The figure shows three views and two pictorial views of one solid part (mm, origin at its lowest corner). Answer the questions. A direction names the side the tool comes from. Coordinates: 2 decimals unless noted, no trailing zeros. Loops run counter-clockwise (first coordinate to the right, second up) from the corner with the lowest first, then second, coordinate; pieces in that order, holes last. Notation, with made-up numbers: M 60,9 L 108,9 A11 cw 108,30 Z; hole C 88,14.25 d4. An arc over 180 degrees is marked long. Answer as a JSON object with one key per item and string values. Group by question number.
1. Given pin 1 (5 mm diameter, centred on y = 39.05, z = 13.5, fed in from -X); pin 2 (1.8 mm diameter, centred on y = 43.05, z = 13.5, fed in from +X); pin 3 (3 mm diameter, centred on x = 5, z = 5.5, fed in from -Y), each flat-ended and moving along its own axis, determine where each tip first touches the part or whether it passes through.
2. A cutting plane is placed at D-D on x = 0.65. State how many separate pieces and enclosed holes the cut face has.
3. Determine the mould class of the marked faces 4, 5 and 6 for opening direction Y: released by +Y, released by -Y, zero draft, split by the parting line, or undercut.
4. A cutting plane is placed at B-B on y = 9.5. Give the vertices of the cut face in (x, z).
5. Straight lines are drawn through the part: L1, parallel to Z at x = 3.55, y = 14; L2, parallel to Y at x = 1.25, z = 6.25; L3, parallel to Z at x = 2.3, y = 20.5 (1 decimal). For each, find the intervals that lie inside material, in ascending order.
6. For the marked faces 1, 2 and 3, determine the directions among +Z, -Z, +X, -X, +Y, -Y from which every point of the face is accessible in a straight line to the end or side of a thin tool.
7. A cutting plane is placed at C-C on z = 13.5. Give the vertices of the cut face in (x, y).
8. A cutting plane is placed at A-A on z = 17.5. Give the vertices of the cut face in (x, y), and give its area (3 significant figures).
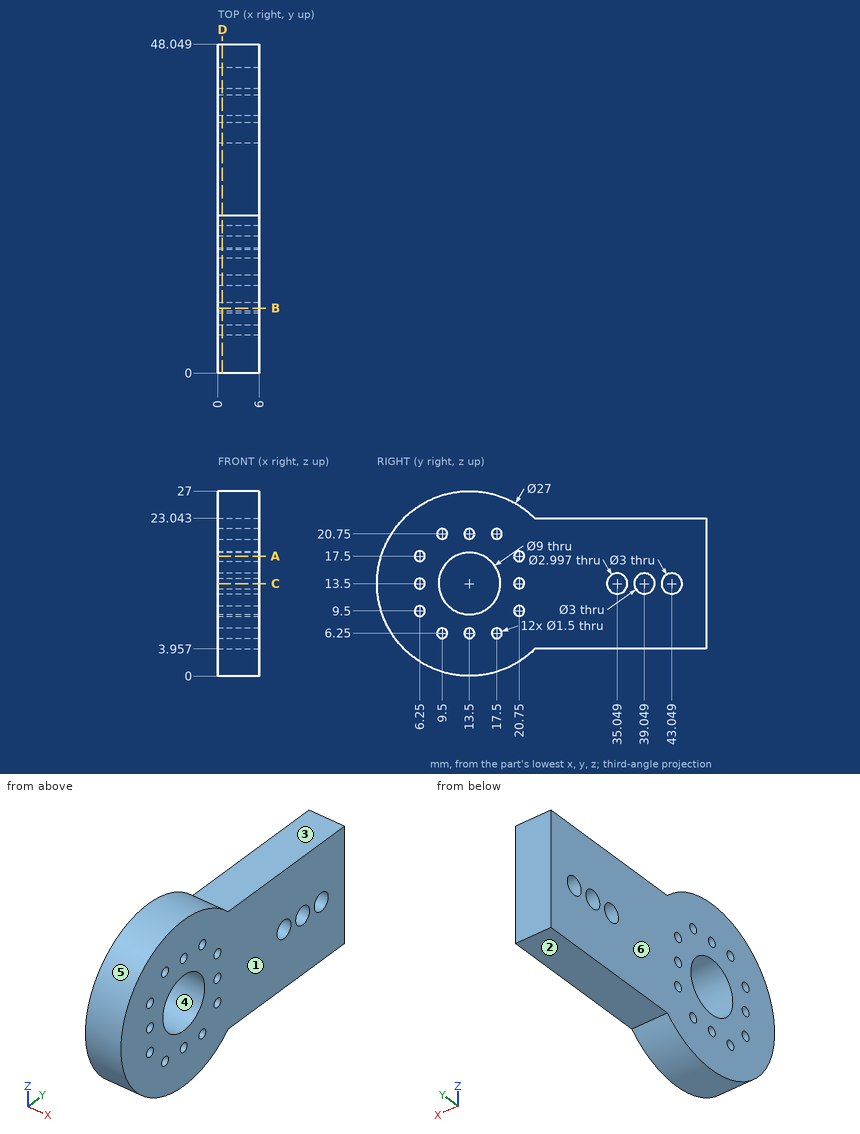
From the geometry:
{
 "1": {"pin 1": "stops at x = 0", "pin 2": "passes through", "pin 3": "stops at y = 1.67"},
 "2": {"separate pieces": "1", "enclosed holes": "16"},
 "3": {"face 4": "undercut", "face 5": "split by the parting line", "face 6": "zero draft"},
 "4": {"outline": "M 0,0.61 L 6,0.61 L 6,5.5 L 0,5.5 Z; M 0,7 L 6,7 L 6,11.44 L 0,11.44 Z; M 0,15.56 L 6,15.56 L 6,20 L 0,20 Z; M 0,21.5 L 6,21.5 L 6,26.39 L 0,26.39 Z"},
 "5": {"L1": "z = 0.01 to 5.69, 6.81 to 9.03, 17.97 to 20.19, 21.31 to 26.99", "L2": "y = 2.11 to 8.75, 10.25 to 12.75, 14.25 to 16.75, 18.25 to 48.05", "L3": "z = 2 to 8.8, 10.2 to 12.8, 14.2 to 16.8, 18.2 to 25"},
 "6": {"face 1": "+Z, -Z, +X, +Y, -Y", "face 2": "-Z, +X, -X, +Y", "face 3": "+Z, +X, -X, +Y"},
 "7": {"outline": "M 0,0 L 6,0 L 6,5.5 L 0,5.5 Z; M 0,7 L 6,7 L 6,9 L 0,9 Z; M 0,18 L 6,18 L 6,20 L 0,20 Z; M 0,21.5 L 6,21.5 L 6,33.55 L 0,33.55 Z; M 0,36.55 L 6,36.55 L 6,37.55 L 0,37.55 Z; M 0,40.55 L 6,40.55 L 6,41.55 L 0,41.55 Z; M 0,44.55 L 6,44.55 L 6,48.05 L 0,48.05 Z"},
 "8": {"outline": "M 0,0.61 L 6,0.61 L 6,5.5 L 0,5.5 Z; M 0,7 L 6,7 L 6,11.44 L 0,11.44 Z; M 0,15.56 L 6,15.56 L 6,20 L 0,20 Z; M 0,21.5 L 6,21.5 L 6,48.05 L 0,48.05 Z", "area": "242 mm²"}
}
